Geometry check sheet. Reference: the model listing, model coordinates, mm. Face numbers are marked on the shaded views. A direction names the side the tool comes from. Give positions to 0.01 mm unless a question says otherwise; leave off trailing zeros. Write each loop counter-clockwise with the first axis right and the second up, starting at its lowest first coordinate (ties: lowest second). Pieces come first, ordered by that corner, then holes. Notation, with made-up numbers: M 78.5,-31.5 L 115.5,-31.5 A10 cw 115.5,-12.5 Z; hole C -17,-39 d7. An arc over 180 degrees is marked long. One line per item, written item: value. Start each with the question number.
1. Scan lines: line 1 (Y direction, x = 13, z = -6); line 2 (X direction, y = -13, z = -2.5); line 3 (X direction, y = -7, z = 18.5). Record each from-to range of solid material in increasing order.
2. Cross-section at D-D on z = 7. Record the cut outline in (x, y), then the cut area to 3 significant figures.
3. Tool access check on the marked faces 4, 5 and 6. Record the directions out of +Z, -Z, +X, -X, +Y, -Y that give a thin tool (end or side, any length) a straight path to the whole face; none if there is none.
4. Cross-section at C-C on y = -2. Record the cut outline in (x, z), then the cut area to 3 significant figures.
5. Gauge pin test, flat ends, axial feed: pin 1 (6 mm diameter, centred on x = 9, y = 14, fed in from -Z); pin 2 (14.5 mm diameter, centred on x = 8, z = 6.5, fed in from -Y); pin 3 (3.5 mm diameter, centred on y = -10.5, z = -9.5, fed in from -X). Record the tip position at first contact, or that the pin passes through.
6. Cross-section at B-B on x = 0. Record the cut outline in (y, z), then the cut area to 3 significant figures.
7. Cross-section at A-A on z = -11. Record the cut outline in (x, y), then the cut area to 3 significant figures.
8. Release check for a two-part mould opening along Y. For the marked faces 1, 2 and 3 record: pulls with the +Y half, pulls with the -Y half, needs draft (parallel to the pull), parting line crosses it, or undercut.
Autodesk Inventor part; units mm, degrees
ref_plane "YZ Plane" through (0, 0, 0) normal (1, 0, 0) x (0, 1, 0)
ref_plane "XZ Plane" through (0, 0, 0) normal (0, 1, 0) x (-1, 0, 0)
ref_plane "XY Plane" through (0, 0, 0) normal (0, 0, 1) x (1, 0, 0)
sketch "Sketch1" plane through (0, 0, 0) normal (0, 0, 1) x (1, 0, 0)
  circle A0 centre (0, 0) radius 23.6793
extrude "Extrusion1" add sketch "Sketch1" along normal blind 10
sketch "Sketch2" plane through (0, 0, 10) normal (0, 0, 1) x (1, 0, 0)
  circle A0 centre (0, 0) radius 21.0238
extrude "Extrusion2" add sketch "Sketch2" along normal blind 12
sketch "Sketch3" plane through (0, 0, 0) normal (0, 0, -1) x (-1, 0, 0)
  line L0 (-16, -5) -> (-1, -5)
  line L1 (-1, -5) -> (-1, -16)
  line L2 (-1, -16) -> (-16, -16)
  line L3 (-16, -16) -> (-16, -5)
  point P0 (0, 0)
extrude "Extrusion3" add sketch "Sketch3" along normal blind 20
sketch "Sketch4" plane through (0, 0, -20) normal (0, 0, -1) x (-1, 0, 0)
  line L0 (-15, -6) -> (-2, -6)
  line L1 (-2, -6) -> (-2, -15)
  line L2 (-2, -15) -> (-15, -15)
  line L3 (-15, -15) -> (-15, -6)
  point P0 (0, 0)
extrude "Extrusion4" cut sketch "Sketch4" against normal through all
sketch "Sketch5" plane through (0, 0, -20) normal (0, 0, -1) x (-1, 0, 0)
  point P0 (0, 0)
properties part number "lid"
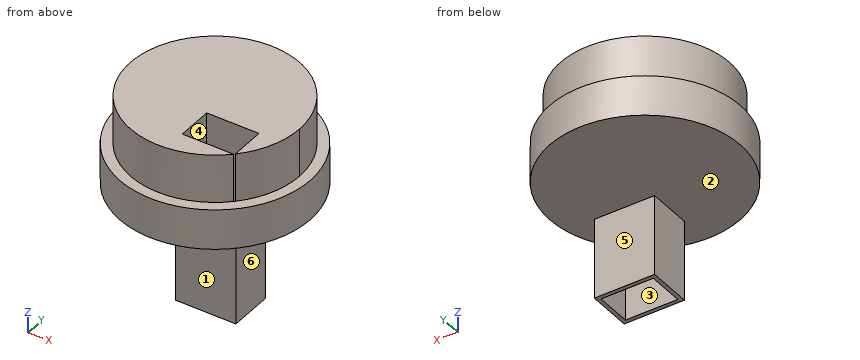
Report:
1. line 1: y = -16 to -15, -6 to -5
1. line 2: x = 1 to 2, 15 to 16
1. line 3: x = -19.82 to 2, 15 to 19.82
2. outline: C 0,0 d47.36; hole M 2,-15 L 15,-15 L 15,-6 L 2,-6 Z
2. area: 1,640 mm^2
3. face 4: +Z, -Z
3. face 5: -Z, +X, -X, +Y
3. face 6: -Z, +X, +Y, -Y
4. outline: M -23.59,0 L 23.59,0 L 23.59,10 L 20.93,10 L 20.93,22 L -20.93,22 L -20.93,10 L -23.59,10 Z
4. area: 974 mm^2
5. pin 1: stops at z = 0
5. pin 2: stops at y = -23.67
5. pin 3: stops at x = 1
6. outline: M -23.68,0 L 23.68,0 L 23.68,10 L 21.02,10 L 21.02,22 L -21.02,22 L -21.02,10 L -23.68,10 Z
6. area: 978 mm^2
7. outline: M 1,-16 L 16,-16 L 16,-5 L 1,-5 Z; hole M 2,-15 L 15,-15 L 15,-6 L 2,-6 Z
7. area: 48.0 mm^2
8. face 1: pulls with the -Y half
8. face 2: needs draft
8. face 3: undercut
